from build123d import *

# Parameters (mm, degrees)
F3_D     = 2.2606
F3_DEPTH = 14.6304
F3_TIP   = 0.6791527577


with BuildPart() as f1:
    # F0 (on Top) → F1 (revolve)
    with BuildSketch(Plane.XY):
        Polygon((0, 25.4), (0, 0), (3.175, 0), (3.175, 6.35), (7.62, 6.35), (7.62, 8.128), align=None)
    revolve(axis=Axis((0, 12.7, 0), (0, 1, 0)))

    # F3
    with Locations(Plane.XZ):
        with Locations((0, 0)):
            Hole(F3_D / 2, depth=F3_DEPTH)
            with Locations((0, 0, -(F3_DEPTH + F3_TIP / 2))):  # 118° drill point
                Cone(0, F3_D / 2, F3_TIP, mode=Mode.SUBTRACT)


solid = f1.part
Can you work these out from the model? Positions are in its coordinate system, mm. A direction names the side the tool comes from. Round coordinates to 2 decimals unless told otherwise and drop trailing zeros. Order: outer loops, then holes, each group sorted by start corner. A loop starts at its lowest first (then second) coordinate and runs counter-clockwise, first axis right, second up. Notation, with made-up numbers: (50, -7.5) -> (55, -7.5) arc R13 ccw to (55, -2.5) -> close; hole circle Ø3 at (-39, 57.25). An arc over 180 degrees is marked (long way). Write each question's results on one line, items separated by ' | '. Start each with the question number.
Item 1: Please list where these lines run through material, in increasing order: L1, parallel to Z at x = 0, y = 6.25 (3 decimals); L2, parallel to Z at x = 0, y = 6.5.
Item 2: Thinking about a two-plate mould opening in Z: for faces 3 (the cylindrical face through (-1.65, 7.25, 7.44)), 4 (the flat face through (-2, 6.35, 3)), 5 (the cylindrical face through (0.245, 7.418, -1.103)), which applies, +Z half, -Z half, draft (parallel to the pull), parting line (faces both ways), or undercut?
Item 3: Which directions (+Z, -Z, +X, -X, +Y, -Y) give clear straight access to the entire face, cutting with the end or side of a thin tool? Please do faces 1 (the flat face through (-1.4, 0, 0)), 2 (the cylindrical face through (-0.69, 3.22, 3.1)).
Item 4: Will these pins go through, and if not, where does the flat tip stop? pin 1 (1.5 mm diameter, centred on x = -3.5, y = 14, fed in from +Z); pin 2 (5 mm diameter, centred on y = 10.5, z = -6, fed in from +X); pin 3 (4 mm diameter, centred on y = 21, z = 2, fed in from +X).
Item 5: If we section it at A-A, the plane y = 18.5: Write out the boundary of the cut face in (x, z).
Results:
1) L1: z = -3.175 to -1.13, 1.13 to 3.175 | L2: z = -7.62 to -1.13, 1.13 to 7.62
2) face 3: parting line | face 4: draft | face 5: undercut
3) face 1: +Z, -Z, +X, -X, -Y | face 2: -Y
4) pin 1: stops at z = 4.35 | pin 2: stops at x = 6.03 | pin 3: stops at x = 2.52
5) outline: circle Ø6.09 at (0, 0)
